from build123d import *

# Parameters (mm, degrees)
SKETCH1_R           = 3.2639
SKETCH1_R_2         = 1.5875
BOSS_EXTRUDE1_DEPTH = 4.7625
SKETCH3_R           = 1.397
CUT_EXTRUDE1_DEPTH  = 6.35
CIRPATTERN1_COUNT   = 3


with BuildPart() as part:
    # Sketch1 → Boss-Extrude1 (new, symmetric)
    with BuildSketch(Plane(origin=(0, 0, 0), x_dir=(1, 0, 0), z_dir=(0, 1, 0))):
        with BuildLine():
            Line((-3.2639, -67.647177805), (-3.2639, -72.952022465))
            ThreePointArc((-3.2639, -72.952022465), (0, -73.025), (3.2639, -72.952022465))
            Line((3.2639, -72.952022465), (3.2639, -67.647177805))
            ThreePointArc((3.2639, -67.647177805), (3.530041907, -66.711459307), (4.248792135, -66.055868937))
            ThreePointArc((4.248792135, -66.055868937), (8.372836069, -62.072061677), (9.46261108, -56.442599084))
            ThreePointArc((9.46261108, -56.442599084), (9.488028557, -55.87828858), (9.68917198, -55.350430914))
            Line((9.68917198, -55.350430914), (52.779465272, 19.28414638))
            ThreePointArc((52.779465272, 19.28414638), (53.136031709, 19.722270528), (53.612030203, 20.026437961))
            ThreePointArc((53.612030203, 20.026437961), (57.942400312, 23.784942101), (59.330456636, 29.348372544))
            ThreePointArc((59.330456636, 29.348372544), (59.538839437, 30.298623685), (60.216124474, 30.996968587))
            Line((60.216124474, 30.996968587), (64.810254712, 33.649390917))
            ThreePointArc((64.810254712, 33.649390917), (63.241505111, 36.5125), (61.546354712, 39.302631548))
            Line((61.546354712, 39.302631548), (56.952224474, 36.650209218))
            ThreePointArc((56.952224474, 36.650209218), (56.00879753, 36.412835622), (55.081664501, 36.707496393))
            ThreePointArc((55.081664501, 36.707496393), (49.569564243, 38.287119576), (44.149419123, 36.416161123))
            ThreePointArc((44.149419123, 36.416161123), (43.648003152, 36.156018052), (43.090293292, 36.066284533))
            Line((43.090293292, 36.066284533), (-43.090293292, 36.066284533))
            ThreePointArc((-43.090293292, 36.066284533), (-43.648003152, 36.156018052), (-44.149419123, 36.416161123))
            ThreePointArc((-44.149419123, 36.416161123), (-49.569564243, 38.287119576), (-55.081664501, 36.707496393))
            ThreePointArc((-55.081664501, 36.707496393), (-56.00879753, 36.412835622), (-56.952224474, 36.650209218))
            Line((-56.952224474, 36.650209218), (-61.546354712, 39.302631548))
            ThreePointArc((-61.546354712, 39.302631548), (-63.241505111, 36.5125), (-64.810254712, 33.649390917))
            Line((-64.810254712, 33.649390917), (-60.216124474, 30.996968587))
            ThreePointArc((-60.216124474, 30.996968587), (-59.538839437, 30.298623685), (-59.330456636, 29.348372544))
            ThreePointArc((-59.330456636, 29.348372544), (-57.942400312, 23.784942101), (-53.612030203, 20.026437961))
            ThreePointArc((-53.612030203, 20.026437961), (-53.136031709, 19.722270528), (-52.779465272, 19.28414638))
            Line((-52.779465272, 19.28414638), (-9.68917198, -55.350430914))
            ThreePointArc((-9.68917198, -55.350430914), (-9.488028557, -55.87828858), (-9.46261108, -56.442599084))
            ThreePointArc((-9.46261108, -56.442599084), (-8.372836069, -62.072061677), (-4.248792135, -66.055868937))
            ThreePointArc((-4.248792135, -66.055868937), (-3.530041907, -66.711459307), (-3.2639, -67.647177805))
        make_face()
        with Locations(Location((0, -57.531, 0), (0, 0, 90))):
            Circle(SKETCH1_R, mode=Mode.SUBTRACT)
        with Locations(Location((-49.823307505, 28.7655, 0), (0, 0, 90))):
            Circle(SKETCH1_R, mode=Mode.SUBTRACT)
        with Locations(Location((49.823307505, 28.7655, 0), (0, 0, 90))):
            Circle(SKETCH1_R, mode=Mode.SUBTRACT)
        with Locations(Location((0, 0, 0), (0, 0, 90))):
            Circle(SKETCH1_R_2, mode=Mode.SUBTRACT)
        with BuildLine():
            Line((3.2639, -41.947085229), (3.2639, -29.931318938))
            ThreePointArc((3.2639, -29.931318938), (3.684254787, -28.783240772), (4.746558577, -28.178019921))
            ThreePointArc((4.746558577, -28.178019921), (8.86834191, -27.164004432), (12.794439011, -25.550595989))
            ThreePointArc((12.794439011, -25.550595989), (14.884524009, -25.921032832), (15.130330606, -28.029410851))
            Line((15.130330606, -28.029410851), (6.581693168, -42.836085229))
            ThreePointArc((6.581693168, -42.836085229), (4.581719738, -43.664501348), (3.2639, -41.947085229))
        make_face(mode=Mode.SUBTRACT)
        with BuildLine():
            Line((-3.2639, -41.947085229), (-3.2639, -29.931318938))
            ThreePointArc((-3.2639, -29.931318938), (-3.684254787, -28.783240772), (-4.746558577, -28.178019921))
            ThreePointArc((-4.746558577, -28.178019921), (-8.86834191, -27.164004432), (-12.794439011, -25.550595989))
            ThreePointArc((-12.794439011, -25.550595989), (-14.884524009, -25.921032832), (-15.130330606, -28.029410851))
            Line((-15.130330606, -28.029410851), (-6.581693168, -42.836085229))
            ThreePointArc((-6.581693168, -42.836085229), (-4.581719738, -43.664501348), (-3.2639, -41.947085229))
        make_face(mode=Mode.SUBTRACT)
        with BuildLine():
            Line((-34.695291423, 23.80016293), (-24.289332569, 17.792279785))
            ThreePointArc((-24.289332569, 17.792279785), (-23.084890319, 17.582278626), (-22.029601791, 18.199650269))
            ThreePointArc((-22.029601791, 18.199650269), (-19.090546952, 21.262211599), (-15.730245703, 23.855607205))
            ThreePointArc((-15.730245703, 23.855607205), (-15.00601092, 25.850892331), (-16.709016547, 27.117956098))
            Line((-16.709016547, 27.117956098), (-33.806291423, 27.117956098))
            ThreePointArc((-33.806291423, 27.117956098), (-35.523707542, 25.80013636), (-34.695291423, 23.80016293))
        make_face(mode=Mode.SUBTRACT)
        with BuildLine():
            Line((-37.959191423, 18.146922299), (-27.553232569, 12.139039154))
            ThreePointArc((-27.553232569, 12.139039154), (-26.769145106, 11.200962147), (-26.776160369, 9.978369652))
            ThreePointArc((-26.776160369, 9.978369652), (-27.958888861, 5.901792833), (-28.524684714, 1.694988784))
            ThreePointArc((-28.524684714, 1.694988784), (-29.890534929, 0.070140501), (-31.839347153, 0.911454753))
            Line((-31.839347153, 0.911454753), (-40.387984591, 15.718129131))
            ThreePointArc((-40.387984591, 15.718129131), (-40.10542728, 17.864364988), (-37.959191423, 18.146922299))
        make_face(mode=Mode.SUBTRACT)
        with BuildLine():
            Line((37.959191423, 18.146922299), (27.553232569, 12.139039154))
            ThreePointArc((27.553232569, 12.139039154), (26.769145106, 11.200962147), (26.776160369, 9.978369652))
            ThreePointArc((26.776160369, 9.978369652), (27.958888861, 5.901792833), (28.524684714, 1.694988784))
            ThreePointArc((28.524684714, 1.694988784), (29.890534929, 0.070140501), (31.839347153, 0.911454753))
            Line((31.839347153, 0.911454753), (40.387984591, 15.718129131))
            ThreePointArc((40.387984591, 15.718129131), (40.10542728, 17.864364988), (37.959191423, 18.146922299))
        make_face(mode=Mode.SUBTRACT)
        with BuildLine():
            Line((34.695291423, 23.80016293), (24.289332569, 17.792279785))
            ThreePointArc((24.289332569, 17.792279785), (23.084890319, 17.582278626), (22.029601791, 18.199650269))
            ThreePointArc((22.029601791, 18.199650269), (19.090546952, 21.262211599), (15.730245703, 23.855607205))
            ThreePointArc((15.730245703, 23.855607205), (15.00601092, 25.850892331), (16.709016547, 27.117956098))
            Line((16.709016547, 27.117956098), (33.806291423, 27.117956098))
            ThreePointArc((33.806291423, 27.117956098), (35.523707542, 25.80013636), (34.695291423, 23.80016293))
        make_face(mode=Mode.SUBTRACT)
    extrude(amount=BOSS_EXTRUDE1_DEPTH, both=True)

    # Sketch3 → Cut-Extrude1 (cut)
    with BuildSketch(Plane.XY.offset(73.025)):
        Circle(SKETCH3_R)
    cut_extrude1 = extrude(amount=-CUT_EXTRUDE1_DEPTH, mode=Mode.SUBTRACT)

    # CirPattern1: Cut-Extrude1 ×3 about axis
    cirpattern1_axis = Axis((0, 0, 0), (0, 1, 0))
    for i in range(1, CIRPATTERN1_COUNT):
        add(cut_extrude1.rotate(cirpattern1_axis, i * 360 / CIRPATTERN1_COUNT), mode=Mode.SUBTRACT)


solid = part.part
The listing builds one solid part. Answer for the finished solid, in the listing's coordinates (mm). A direction names the side the tool comes from. Give positions to 0.01 mm unless a question says otherwise; leave off trailing zeros. Write each loop counter-clockwise with the first axis right and the second up, starting at its lowest first coordinate (ties: lowest second). Pieces come first, ordered by that corner, then holes. Notation, with made-up numbers: (34.25, -23) -> (75.25, -23) arc R32 cw to (75.25, 11) -> close; hole circle Ø1 at (33.25, 17). An arc over 180 degrees is marked (long way). Use a Markdown table: item, result.
(1) Section A-A, the plane x = 0 is taken. Determine the outline of the cut face in (y, z) (1 decimal).
Return value:
| item | result |
|---|---|
| outline | (-4.8, -36.1) -> (4.8, -36.1) -> (4.8, -1.6) -> (-4.8, -1.6) -> close; (-4.8, 1.6) -> (4.8, 1.6) -> (4.8, 54.3) -> (-4.8, 54.3) -> close; (-4.8, 60.8) -> (4.8, 60.8) -> (4.8, 73) -> (1.4, 73) -> (1.4, 66.7) -> (-1.4, 66.7) -> (-1.4, 73) -> (-4.8, 73) -> close |
(2) Section B-B, the plane y = 0 is taken. Give the number of separate pieces and of enclosed holes in the cut face, then the cut area to 3 significant figures.
Return value:
| item | result |
|---|---|
| separate pieces | 1 |
| enclosed holes | 10 |
| area | 6,020 mm2 |
(3) Section D-D, the plane z = 18.5 is taken. Determine the outline of the cut face in (x, y).
Return value:
| item | result |
|---|---|
| outline | (-30.96, -4.76) -> (30.96, -4.76) -> (30.96, 4.76) -> (-30.96, 4.76) -> close |
(4) Find the intervals of material crossed by probe 1 along Y at (x, z) = (0, 69.5); probe 2 along X at (y, z) = (0, 69); probe 3 along X at (y, z) = (-0.75, 45.5), in increasing order. Write a range as from..to.
Return value:
| item | result |
|---|---|
| probe 1 | -4.76..-1.4, 1.4..4.76 |
| probe 2 | -3.26..-1.4, 1.4..3.26 |
| probe 3 | -15.38..15.38 |
(5) Determine the mould class of faces 4 (the flat face through (0, 0, 66.675)), 5 (the flat face through (29.57, -0.07, -20.84)) for opening direction Y: released by +Y, released by -Y, zero draft, split by the parting line, or undercut.
Return value:
| item | result |
|---|---|
| face 4 | undercut |
| face 5 | zero draft |
(6) Flat-ended cylindrical pins translate along their axes: P1, Ø4, axis at x = 50.5, y = 3, coming from the -Z side; P2, Ø4.5, axis at x = 0, y = 0, coming from the -Z side; P3, Ø1, axis at y = 3, z = 47.5, coming from the -X side; P4, Ø6, axis at x = 0, z = 57.531, coming from the +Y side. Find the tip coordinate at first contact, or state that the pin passes through.
Return value:
| item | result |
|---|---|
| P1 | z = -38.29 |
| P2 | z = -36.07 |
| P3 | x = -14.51 |
| P4 | through |
(7) For faces 1 (the flat face through (-31.536, 0.067, 17.511)), 2 (the flat face through (-25, 0, -27.118)), 3 (the flat face through (-59.22, 0.07, -37.96)), determine the directions among +Z, -Z, +X, -X, +Y, -Y from which every point of the face is accessible in a straight line to the end or side of a thin tool.
Return value:
| item | result |
|---|---|
| face 1 | +Z, -X, +Y, -Y |
| face 2 | +Y, -Y |
| face 3 | -Z, +Y, -Y |
(8) Section C-C, the plane z = 46.5 is taken. Determine the outline of the cut face in (x, y).
Return value:
| item | result |
|---|---|
| outline | (-14.8, -4.76) -> (14.8, -4.76) -> (14.8, 4.76) -> (-14.8, 4.76) -> close |
